CAD build for the part. Positions are in the model's coordinates, mm. A direction names the side the tool comes from. Round coordinates to 2 decimals unless told otherwise and drop trailing zeros. Order: outer loops, then holes, each group sorted by start corner. A loop starts at its lowest first (then second) coordinate and runs counter-clockwise, first axis right, second up. Notation, with made-up numbers: M 58,73 L 100,73 A11 cw 100,83 Z; hole C -35.5,-15.5 d6. An arc over 180 degrees is marked long. Answer as a JSON object with one key per item and string values. Group by question number.
```python
from build123d import *
from build123d.topology import SkipClean

# Parameters (mm, degrees)
EXTRUDE_1_DEPTH      = 5
EXTRUDE_1_DEPTH_BACK = 50
SKETCH_2_R           = 2.1
CUT_EXTRUDE_1_DEPTH  = 56.722526863
SKETCH_13_R          = 8.470611641
CUT_EXTRUDE_6_DEPTH  = 5
EXTRUDE_START        = 8
EXTRUDE_4_DEPTH      = 8
SKETCH_18_R          = 3.1
CUT_EXTRUDE_7_DEPTH  = 3.05
EXTRUDE_5_DEPTH      = 8
SKETCH_21_W          = 70
SKETCH_21_H          = 8
EXTRUDE_6_DEPTH      = 60
SKETCH_22_W          = 64
SKETCH_22_H          = 54
CUT_EXTRUDE_8_DEPTH  = 5


with BuildPart() as part:
    # ｽｹｯﾁ1 → ﾎﾞｽ - 押し出し1 (new, two sides: drawn at the far end of the back side and taken through both)
    with BuildSketch(Plane.XY.offset(-EXTRUDE_1_DEPTH_BACK)):
        with BuildLine():
            Line((3.464101615, 2), (8, 2))
            Line((8, 2), (8, -2))
            Line((8, -2), (3.464101615, -2))
            ThreePointArc((3.464101615, -2), (-4, 0), (3.464101615, 2))
        make_face()
    extrude(amount=EXTRUDE_1_DEPTH + EXTRUDE_1_DEPTH_BACK)

    # ｽｹｯﾁ2 → ｶｯﾄ - 押し出し1 (cut, through all)
    with BuildSketch(Plane(origin=(0, 0, -50), x_dir=(-1, 0, 0), z_dir=(0, 0, -1))):
        Circle(SKETCH_2_R)
    extrude(amount=-CUT_EXTRUDE_1_DEPTH, mode=Mode.SUBTRACT)

    # ｽｹｯﾁ13 → ｶｯﾄ - 押し出し6 (cut)
    with BuildSketch(Plane.XY.offset(5)):
        Circle(SKETCH_13_R)
    extrude(amount=-CUT_EXTRUDE_6_DEPTH, mode=Mode.SUBTRACT)

    # ｽｹｯﾁ15 → ﾎﾞｽ - 押し出し4 (add)
    with SkipClean():  # the faces are left unmerged after this step: merging them gives an invalid solid
        with BuildSketch(Plane(origin=(0, 0, -50), x_dir=(-1, 0, 0), z_dir=(0, 0, -1)).offset(EXTRUDE_START)):
            with BuildLine():
                Line((40, -4), (0, -4))
                ThreePointArc((0, -4), (-4, 0), (0, 4))
                Line((0, 4), (40, 4))
                ThreePointArc((40, 4), (44, 0), (40, -4))
            make_face()
        extrude(amount=-EXTRUDE_4_DEPTH)

    # ｽｹｯﾁ18 → ｶｯﾄ - 押し出し7 (cut)
    with SkipClean():  # the faces are left unmerged after this step: merging them gives an invalid solid
        with BuildSketch(Plane(origin=(0, 0, -58), x_dir=(-1, 0, 0), z_dir=(0, 0, -1))):
            Circle(SKETCH_18_R)
            with Locations((40, 0)):
                Circle(SKETCH_18_R)
            with Locations((20, 0)):
                Circle(SKETCH_18_R)
            with Locations((10, 0)):
                Circle(SKETCH_18_R)
            with Locations((30, 0)):
                Circle(SKETCH_18_R)
        extrude(amount=-CUT_EXTRUDE_7_DEPTH, mode=Mode.SUBTRACT)

    # ｽｹｯﾁ20 → ﾎﾞｽ - 押し出し5 (add)
    with BuildSketch(Plane(origin=(0, 0, -50), x_dir=(-1, 0, 0), z_dir=(0, 0, -1)).offset(EXTRUDE_START)):
        with BuildLine():
            Line((-3.464101615, 2), (-8, 2))
            Line((-8, 2), (-8, -2))
            Line((-8, -2), (-3.464101615, -2))
            ThreePointArc((-3.464101615, -2), (-4, 0), (-3.464101615, 2))
        make_face()
    extrude(amount=-EXTRUDE_5_DEPTH)

    # ｽｹｯﾁ21 → ﾎﾞｽ - 押し出し6 (add)
    with BuildSketch(Plane.XY):
        with Locations((-27, 0)):
            Rectangle(SKETCH_21_W, SKETCH_21_H)
    extrude(amount=EXTRUDE_6_DEPTH)

    # ｽｹｯﾁ22 → ｶｯﾄ - 押し出し8 (cut)
    with BuildSketch(Plane(origin=(0, 4, 0), x_dir=(1, 0, 0), z_dir=(0, 1, 0))):
        with Locations((-27, -30)):
            Rectangle(SKETCH_22_W, SKETCH_22_H)
    extrude(amount=-CUT_EXTRUDE_8_DEPTH, mode=Mode.SUBTRACT)


solid = part.part
```
Item 1: Cut at A-A, the plane x = -20. Give the cut face in (y, z).
Item 2: Flat gauge pins, fed straight in: pin 1 Ø1.4 at (x, z) = (7, -18) entering from -Y; pin 2 Ø3 at (x, y) = (-41, 0.5) entering from -Z; pin 3 Ø6 at (x, z) = (-50, 46) entering from +Y. Where does each tip first touch, or does it go through?
Item 3: Two-plate mould, pull along X, no slides. Class faces 1 (the face through (8, 0, 13)), 2 (the face through (-26.9, 0.1, -56.5)), 3 (the face through (-27, 0, 60)): +X half, -X half, draft (parallel to the pull), parting line (faces both ways), or undercut.
Item 4: 3-axis set-ups, long thin cutter, end or side, ignore diameter. For faces 4 (the face through (-27, 2, 57)), 5 (the face through (0, 0, -50)), 6 (the face through (-30, 0, -54.95)): which of +Z, -Z, +X, -X, +Y, -Y reach the whole face in a straight line?
Item 5: Drill centre lines: line 1 (Z direction, x = -23.5, y = 1); line 2 (Z direction, x = -22, y = -0.5); line 3 (Z direction, x = -37.5, y = -2.75). Where is each one in solid material? Low to high. Write a range as [from, to].
Item 6: Cut at B-B, the plane z = 5. Give the cut face in (x, y).
Response values:
{
 "1": {"outline": "M -4,-58 L -3.1,-58 L -3.1,-54.95 L 3.1,-54.95 L 3.1,-58 L 4,-58 L 4,-50 L -4,-50 Z; M -4,0 L 4,0 L 4,3 L -1,3 L -1,57 L 4,57 L 4,60 L -4,60 Z"},
 "2": {"pin 1": "y = -2", "pin 2": "z = -54.95", "pin 3": "y = -1"},
 "3": {"face 1": "+X half", "face 2": "undercut", "face 3": "draft"},
 "4": {"face 4": "+Y", "face 5": "none", "face 6": "-Z"},
 "5": {"line 1": "[-58, -50], [0, 3], [57, 60]", "line 2": "[-54.95, -50], [0, 3], [57, 60]", "line 3": "[-58, -50], [0, 60]"},
 "6": {"outline": "M -62,-4 L 8,-4 L 8,4 L 5,4 L 5,-1 L -59,-1 L -59,4 L -62,4 Z"}
}
